Geometry: see drawing. Coordinates: mm, zero at the bounding-box minimum. A direction names the side the tool comes from. Round coordinates to 2 decimals unless told otherwise and drop trailing zeros. Order: outer loops, then holes, each group sorted by start corner. A loop starts at its lowest first (then second) coordinate and runs counter-clockwise, first axis right, second up. Notation, with made-up numbers: (-15.5, 20) -> (0.5, 20) arc R18 ccw to (0.5, 49) -> close; hole circle Ø7 at (22, -16.75). An arc over 180 degrees is marked (long way). Put each result on its own line as item: value.
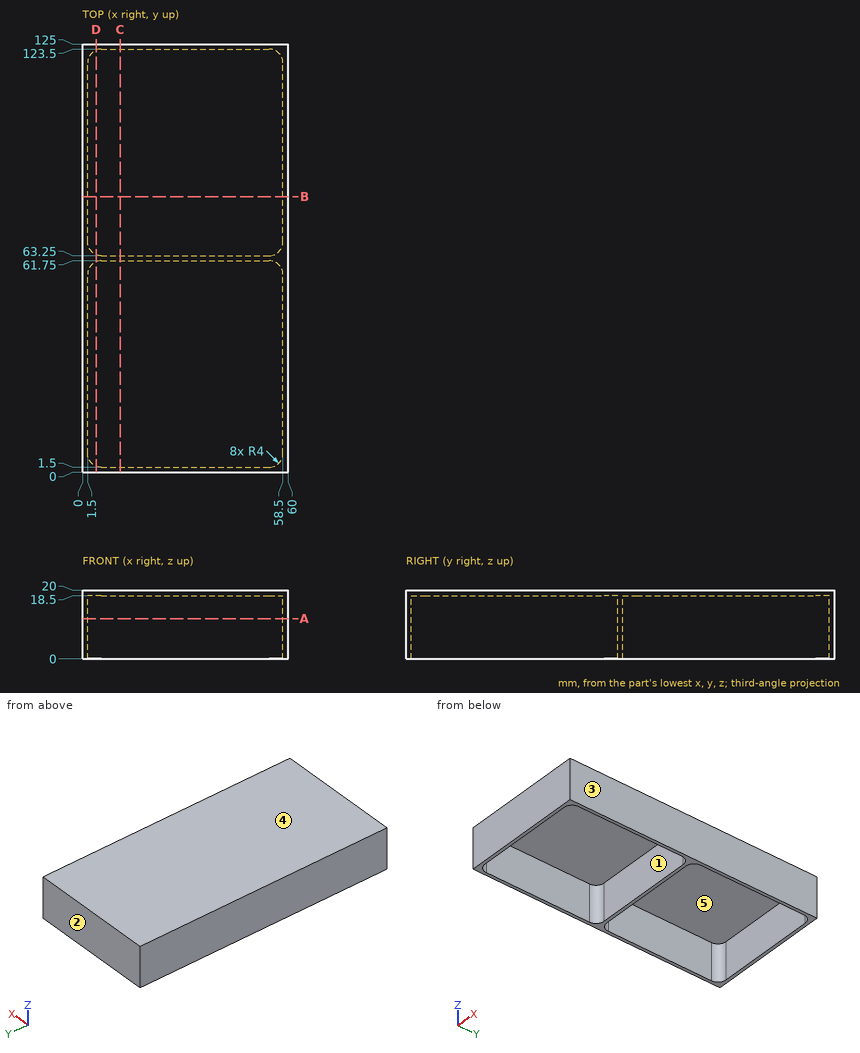
1. Set-up query: the marked faces 1 and 2. Return all of +Z, -Z, +X, -X, +Y, -Y with unobstructed straight access to the full face (end or side cutting, diameter ignored); none if empty.
Ans:
face 1: -Z
face 2: +Z, -Z, +X, -X, +Y
2. Material intervals for probe 1 along Y at (x, z) = (32, 8.75); probe 2 along X at (y, z) = (39, 17.75); probe 3 along Z at (x, y) = (31.5, 11), sorted ascending.
Ans:
probe 1: 0 to 1.5, 61.75 to 63.25, 123.5 to 125
probe 2: 0 to 1.5, 58.5 to 60
probe 3: 18.5 to 20
3. Cut plane D-D on x = 4. Return loops of the section in (y, z), and give its area (3 significant figures).
Ans:
outline: (0, 0) -> (1.79, 0) -> (1.79, 18.5) -> (61.46, 18.5) -> (61.46, 0) -> (63.54, 0) -> (63.54, 18.5) -> (123.21, 18.5) -> (123.21, 0) -> (125, 0) -> (125, 20) -> (0, 20) -> close
area: 292 mm²
4. Contact query for a flat-ended pin moving along its axis: P1, Ø10, axis at x = 11, y = 50, coming from the -Z side. Output: stop coordinate, or through.
Ans:
P1: z = 18.5
5. Draft query along X for the marked faces 3, 4 and 5. Return one class per face: +X half, -X half, draft (parallel to the pull), parting line (faces both ways), or undercut.
Ans:
face 3: +X half
face 4: draft
face 5: undercut
6. Cut plane A-A on z = 11.75. Return loops of the section in (x, y), and give its area (3 significant figures).
Ans:
outline: (0, 0) -> (60, 0) -> (60, 125) -> (0, 125) -> close; hole (1.5, 5.5) arc R4 ccw to (5.5, 1.5) -> (54.5, 1.5) arc R4 ccw to (58.5, 5.5) -> (58.5, 57.75) arc R4 ccw to (54.5, 61.75) -> (5.5, 61.75) arc R4 ccw to (1.5, 57.75) -> close; hole (1.5, 67.25) arc R4 ccw to (5.5, 63.25) -> (54.5, 63.25) arc R4 ccw to (58.5, 67.25) -> (58.5, 119.5) arc R4 ccw to (54.5, 123.5) -> (5.5, 123.5) arc R4 ccw to (1.5, 119.5) -> close
area: 659 mm²
7. Cut plane C-C on x = 11. Return loops of the section in (y, z).
Ans:
outline: (0, 0) -> (1.5, 0) -> (1.5, 18.5) -> (61.75, 18.5) -> (61.75, 0) -> (63.25, 0) -> (63.25, 18.5) -> (123.5, 18.5) -> (123.5, 0) -> (125, 0) -> (125, 20) -> (0, 20) -> close
8. Cut plane B-B on y = 80.5. Return loops of the section in (x, z).
Ans:
outline: (0, 0) -> (1.5, 0) -> (1.5, 18.5) -> (58.5, 18.5) -> (58.5, 0) -> (60, 0) -> (60, 20) -> (0, 20) -> close
